```python
from build123d import *

# Parameters (mm, degrees)
SKETCH1_W           = 50.8
SKETCH1_H           = 50.8
BOSS_EXTRUDE1_DEPTH = 12.7
F_10_CB_D           = 4.826
F_10_CB_CBORE_D     = 6.35
F_10_CB_CBORE_DEPTH = 4.826
F_6_CB_D            = 3.5052
F_6_CB_DEPTH        = 50.8
F_6_CB_CBORE_D      = 6.35
F_6_CB_CBORE_DEPTH  = 3.5052


with BuildPart() as part:
    # Sketch1 → Boss-Extrude1 (new body)
    with BuildSketch(Plane.XY):
        Rectangle(SKETCH1_W, SKETCH1_H)
    extrude(amount=BOSS_EXTRUDE1_DEPTH)

    # #10 CB (through all)
    with Locations(Plane(origin=(0, 0, 0), x_dir=(1, 0, 0), z_dir=(0, 0, -1))):
        with Locations((0, -19.05), (0, 0), (0, 19.05)):
            CounterBoreHole(F_10_CB_D / 2, F_10_CB_CBORE_D / 2, F_10_CB_CBORE_DEPTH)

    # #6 CB
    with Locations(Plane.XY.offset(12.7)):
        with Locations((-9.525, 19.05), (-9.525, -19.05), (9.525, -19.05), (9.525, 19.05)):
            CounterBoreHole(F_6_CB_D / 2, F_6_CB_CBORE_D / 2, F_6_CB_CBORE_DEPTH, depth=F_6_CB_DEPTH)


solid = part.part
```
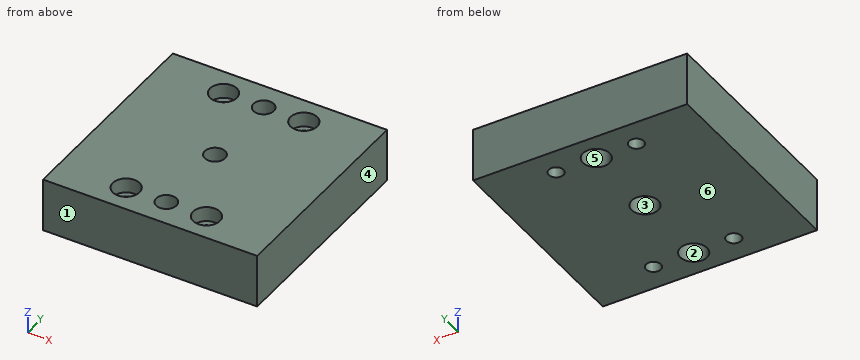
Geometry: final body of the model. Coordinates: model frame, mm. Face numbers are marked on the shaded views. A direction names the side the tool comes from. Coordinates: 2 decimals unless noted, no trailing zeros. Order: outer loops, then holes, each group sorted by start corner. A loop starts at its lowest first (then second) coordinate and runs counter-clockwise, first axis right, second up. Notation, with made-up numbers: M 28.5,-3 L 37.5,-3 A12 cw 37.5,12 Z; hole C 46,73 d9. An arc over 180 degrees is marked long. Answer as CSV lines item,"result".
Q1. Section D-D on y = 0. Return the cut outline in (x, z) (3 decimals), and give its area (3 significant figures).
Answers:
outline,"M -25.4,0 L -3.175,0 L -3.175,4.826 L -2.413,4.826 L -2.413,12.7 L -25.4,12.7 Z; M 2.413,4.826 L 3.175,4.826 L 3.175,0 L 25.4,0 L 25.4,12.7 L 2.413,12.7 Z"
area,"577 mm^2"
Q2. Section A-A on x = 0. Return the cut outline in (y, z) (3 decimals).
Answers:
outline,"M -25.4,0 L -22.225,0 L -22.225,4.826 L -21.463,4.826 L -21.463,12.7 L -25.4,12.7 Z; M -16.637,4.826 L -15.875,4.826 L -15.875,0 L -3.175,0 L -3.175,4.826 L -2.413,4.826 L -2.413,12.7 L -16.637,12.7 Z; M 2.413,4.826 L 3.175,4.826 L 3.175,0 L 15.875,0 L 15.875,4.826 L 16.637,4.826 L 16.637,12.7 L 2.413,12.7 Z; M 21.463,4.826 L 22.225,4.826 L 22.225,0 L 25.4,0 L 25.4,12.7 L 21.463,12.7 Z"
Q3. Line query: probe 1 along Y at (x, z) = (0, 2.7) (3 decimals); probe 2 along X at (y, z) = (19, 5.5); probe 3 along Y at (x, z) = (-2, 7.75). Output: solid intervals per line, ascending. Write a range as [from, to].
Answers:
probe 1,"y = [-25.4, -22.225], [-15.875, -3.175], [3.175, 15.875], [22.225, 25.4]"
probe 2,"x = [-25.4, -11.28], [-7.77, -2.41], [2.41, 7.77], [11.28, 25.4]"
probe 3,"y = [-25.4, -20.4], [-17.7, -1.35], [1.35, 17.7], [20.4, 25.4]"
Q4. Draft query along X for the marked faces 1, 2, 3 and 4. Return one class per face: pulls with the +X half, pulls with the -X half, needs draft (parallel to the pull), parting line crosses it, or undercut.
Answers:
face 1,"needs draft"
face 2,"undercut"
face 3,"undercut"
face 4,"pulls with the +X half"
Q5. Set-up query: the marked faces 5 and 6. Return all of +Z, -Z, +X, -X, +Y, -Y with unobstructed straight access to the full face (end or side cutting, diameter ignored); none if empty.
Answers:
face 5,"-Z"
face 6,"-Z, +X, -X, +Y, -Y"
Q6. First-contact query: P1, Ø1.9, axis at x = -8.5, y = -18, coming from the +Z side; P2, Ø4.5, axis at x = 0, y = -19.05, coming from the -Z side. Flat tips, straight axial feed; report the tip coordinate or a pass-through.
Answers:
P1,"stops at z = 9.19"
P2,"passes through"
Q7. Section B-B on z = 5.75. Return the cut outline in (x, y) (3 decimals).
Answers:
outline,"M -25.4,-25.4 L 25.4,-25.4 L 25.4,25.4 L -25.4,25.4 Z; hole C -9.525,-19.05 d3.505; hole C -9.525,19.05 d3.505; hole C 0,-19.05 d4.826; hole C 0,0 d4.826; hole C 0,19.05 d4.826; hole C 9.525,-19.05 d3.505; hole C 9.525,19.05 d3.505"
Q8. Section C-C on y = -19.05. Return the cut outline in (x, z) (3 decimals), and give its area (3 significant figures).
Answers:
outline,"M -25.4,0 L -11.278,0 L -11.278,9.195 L -12.7,9.195 L -12.7,12.7 L -25.4,12.7 Z; M -7.772,0 L -3.175,0 L -3.175,4.826 L -2.413,4.826 L -2.413,12.7 L -6.35,12.7 L -6.35,9.195 L -7.772,9.195 Z; M 2.413,4.826 L 3.175,4.826 L 3.175,0 L 7.772,0 L 7.772,9.195 L 6.35,9.195 L 6.35,12.7 L 2.413,12.7 Z; M 11.278,0 L 25.4,0 L 25.4,12.7 L 12.7,12.7 L 12.7,9.195 L 11.278,9.195 Z"
area,"468 mm^2"
